```python
from build123d import *

# Parameters (mm, degrees)
F0_R           = 6.35
F1_DEPTH       = 25.4
F2_R           = 6.35
F3_DEPTH       = 13.716
F5_DEPTH       = 7.493
F6_DEPTH       = 5.08
F8_D           = 2.921
F8_CBORE_D     = 4.699
F8_CBORE_DEPTH = 10.922
F9_DEPTH       = 10.922
F10_DEPTH      = 17.907


with BuildPart() as f1:
    # F0 (on Front) → F1 (new body)
    with BuildSketch(Plane.XZ):
        with BuildLine():
            Line((0, -13.589), (17.1026142738, -13.589))
            ThreePointArc((17.1026142738, -13.589), (0, 21.844), (-17.1026142738, -13.589))
            Line((-17.1026142738, -13.589), (0, -13.589))
        make_face()
        Circle(F0_R, mode=Mode.SUBTRACT)
    extrude(amount=F1_DEPTH)

    # F2 (on face) → F3 (cut)
    with BuildSketch(Plane(origin=(0, 0, 0), x_dir=(-1, 0, 0), z_dir=(0, 1, 0))):
        with BuildLine():
            Line((-3.2512, 21.6006952333), (-3.2512, 15.5385109827))
            ThreePointArc((-3.2512, 15.5385109827), (-15.6500961726, 2.6627269459), (-8.2069911661, -13.589))
            Line((-8.2069911661, -13.589), (8.2069911661, -13.589))
            ThreePointArc((8.2069911661, -13.589), (15.6500961726, 2.6627269459), (3.2512, 15.5385109827))
            Line((3.2512, 15.5385109827), (3.2512, 21.6006952333))
            ThreePointArc((3.2512, 21.6006952333), (0, 21.844), (-3.2512, 21.6006952333))
        make_face()
        Circle(F2_R, mode=Mode.SUBTRACT)
    extrude(amount=-F3_DEPTH, mode=Mode.SUBTRACT)

    # F4 (on face) → F5 (cut)
    with BuildSketch(Plane(origin=(0, 0, 0), x_dir=(-1, 0, 0), z_dir=(0, 1, 0))):
        with BuildLine():
            Line((-17.1026142738, -13.589), (-8.2069911661, -13.589))
            ThreePointArc((-8.2069911661, -13.589), (-15.6500961726, 2.6627269459), (-3.2512, 15.5385109827))
            Line((-3.2512, 15.5385109827), (-3.2512, 16.129))
            Line((-3.2512, 16.129), (-14.731452576, 16.129))
            ThreePointArc((-14.731452576, 16.129), (-16.3464246709, 14.4898149222), (-17.78, 12.6898359327))
            Line((-17.78, 12.6898359327), (-17.78, -12.6898359327))
            ThreePointArc((-17.78, -12.6898359327), (-17.44710058, -13.1437824598), (-17.1026142738, -13.589))
        make_face()
        with BuildLine():
            Line((-8.2069911661, -13.589), (0, -13.589))
            Line((0, -13.589), (17.78, -13.589))
            Line((17.78, -13.589), (17.78, 16.129))
            Line((17.78, 16.129), (-3.2512, 16.129))
            Line((-3.2512, 16.129), (-3.2512, 15.5385109827))
            ThreePointArc((-3.2512, 15.5385109827), (-15.6500961726, 2.6627269459), (-8.2069911661, -13.589))
        make_face()
    extrude(amount=-F5_DEPTH, mode=Mode.SUBTRACT)

    # F6 (cut): faces of the model
    f6_faces = [f1.faces().sort_by_distance(p)[0] for p in [
        (7.5018293791, 0, 18.2089166426),
        (-7.5018293791, 0, 18.2089166426),
    ]]
    extrude(f6_faces, amount=-F6_DEPTH, mode=Mode.SUBTRACT)

    # F8 (through all)
    with Locations(Plane.XZ.offset(25.4)):
        with Locations((-14.2875, -9.1525132509), (-14.2875, 12.3104867491), (14.2875, 12.3104867491), (14.2875, -9.1525132509)):
            CounterBoreHole(F8_D / 2, F8_CBORE_D / 2, F8_CBORE_DEPTH)

    # F7 (on face) → F9 (cut)
    with BuildSketch(Plane.XZ.offset(25.4)):
        with BuildLine():
            Line((-12.827, -13.589), (-11.938, -13.589))
            Line((-11.938, -13.589), (-11.938, -9.1525132509))
            ThreePointArc((-11.938, -9.1525132509), (-12.1990496422, -8.0761650949), (-12.9241888511, -7.239))
            Line((-12.9241888511, -7.239), (-13.6989384625, -7.239))
            ThreePointArc((-13.6989384625, -7.239), (-13.8035807397, -7.0374139258), (-13.9052567889, -6.8343155938))
            ThreePointArc((-13.9052567889, -6.8343155938), (-15.8077088385, -7.3611128665), (-16.637, -9.1525132509))
            Line((-16.637, -9.1525132509), (-16.637, -13.589))
            Line((-16.637, -13.589), (-15.748, -13.589))
            Line((-15.748, -13.589), (-15.748, -9.1525132509))
            ThreePointArc((-15.748, -9.1525132509), (-14.2875, -7.6920132509), (-12.827, -9.1525132509))
            Line((-12.827, -9.1525132509), (-12.827, -13.589))
        make_face()
        with BuildLine():
            ThreePointArc((12.827, -9.1525132509), (14.2875, -7.6920132509), (15.748, -9.1525132509))
            Line((15.748, -9.1525132509), (15.748, -13.589))
            Line((15.748, -13.589), (16.637, -13.589))
            Line((16.637, -13.589), (16.637, -9.1525132509))
            ThreePointArc((16.637, -9.1525132509), (15.8077088385, -7.3611128665), (13.9052567889, -6.8343155938))
            ThreePointArc((13.9052567889, -6.8343155938), (13.8035807397, -7.0374139258), (13.6989384625, -7.239))
            Line((13.6989384625, -7.239), (12.9241888511, -7.239))
            ThreePointArc((12.9241888511, -7.239), (12.1990496422, -8.0761650949), (11.938, -9.1525132509))
            Line((11.938, -9.1525132509), (11.938, -13.589))
            Line((11.938, -13.589), (12.827, -13.589))
            Line((12.827, -13.589), (12.827, -9.1525132509))
        make_face()
    extrude(amount=-F9_DEPTH, mode=Mode.SUBTRACT)

    # F7 (on face) → F10 (cut)
    with BuildSketch(Plane.XZ.offset(25.4)):
        with BuildLine():
            Line((-15.748, -13.589), (-12.827, -13.589))
            Line((-12.827, -13.589), (-12.827, -9.1525132509))
            ThreePointArc((-12.827, -9.1525132509), (-14.2875, -7.6920132509), (-15.748, -9.1525132509))
            Line((-15.748, -9.1525132509), (-15.748, -13.589))
        make_face()
        with BuildLine():
            Line((15.748, -13.589), (15.748, -9.1525132509))
            ThreePointArc((15.748, -9.1525132509), (14.2875, -7.6920132509), (12.827, -9.1525132509))
            Line((12.827, -9.1525132509), (12.827, -13.589))
            Line((12.827, -13.589), (15.748, -13.589))
        make_face()
    extrude(amount=-F10_DEPTH, mode=Mode.SUBTRACT)


solid = f1.part
```
The model under review builds one solid part; all positions refer to its coordinate system, in mm. A direction names the side the tool comes from. Round coordinates to 2 decimals unless told otherwise and drop trailing zeros. Loops run counter-clockwise (first coordinate to the right, second up) from the corner with the lowest first, then second, coordinate; pieces in that order, holes last. Notation, with made-up numbers: (-4.5, 17.25) -> (45.5, 17.25) arc R30 cw to (45.5, 55.25) -> close; hole circle Ø1 at (14.25, -30.5). An arc over 180 degrees is marked (long way). Answer as a JSON object with one key per item and string values. Group by question number.
1) For faces 1 (the face through (13, -14.478, 11)), 2 (the face through (12.827, -11, -11)), 3 (the face through (-9, -6, 16.129)), list the 3-axis set-ups (+Z, -Z, +X, -X, +Y, -Y) from which the entire face can be reached by the end or side of a thin tool; tool diameter is ignored.
2) We need section B-B on y = -6.25. Write out the cut boundary in (x, z).
3) Mouldability with a two-part tool opening along X and no side actions: class faces 4 (the face through (-12.75, -14.478, 11.82)), 5 (the face through (19, 0, 0)), 6 (the face through (0.686, -15.344, 21.833)) as released by +X, released by -X, zero draft, split by the parting line, or undercut.
4) We need section D-D on y = -10.5. Give the number of separate pieces and of enclosed holes in the cut face, then the cut area to 3 significant figures.
5) For line 1 (X direction, y = -8.5, z = -11); line 2 (X direction, y = -18.25, z = -8); line 3 (X direction, y = -23.5, z = -9.5), list the stretches that pass through material, from the lowest coordinate up. Write a range as [from, to].
6) We need section A-A on z = 0. Write out the cut boundary in (x, y) (3 decimals).
7) For pin 1 Ø16 at (x, z) = (-2.5, -1.5) entering from +Y; pin 2 Ø6 at (x, z) = (11, 20) entering from +Y; pin 3 Ø4.5 at (x, z) = (-11, -11) entering from +Y, all flat-tipped, find the tip position at first contact; note any pin that passes through.
8) We need section C-C on x = 0. Write out the cut boundary in (y, z), then the cut area to 3 significant figures.
Result set:
{
 "1": {"face 1": "-Y", "face 2": "-Z, +Y, -Y", "face 3": "-Z, +X, -X, +Y"},
 "2": {"outline": "(-17.78, -12.69) -> (-17.78, 12.69) arc R21.84 ccw to start; (-14.73, 16.13) -> (-3.25, 16.13) -> (-3.25, 21.6) arc R21.84 ccw to start; (3.25, 16.13) -> (14.73, 16.13) arc R21.84 ccw to (3.25, 21.6) -> close; (17.78, -12.69) arc R21.84 ccw to (17.78, 12.69) -> close"},
 "3": {"face 4": "undercut", "face 5": "zero draft", "face 6": "split by the parting line"},
 "4": {"separate pieces": "4", "enclosed holes": "2", "area": "452 mm²"},
 "5": {"line 1": "[-18.87, -15.75], [-12.83, -11.45], [11.45, 12.83], [15.75, 18.87]", "line 2": "[-20.33, -16.33], [-12.24, 12.24], [16.33, 20.33]", "line 3": "[-19.67, -16.64], [-11.94, 11.94], [16.64, 19.67]"},
 "6": {"outline": "(-21.844, -25.4) -> (-6.35, -25.4) -> (-6.35, -13.716) -> (-15.875, -13.716) -> (-15.875, -7.493) -> (-17.78, -7.493) -> (-17.78, 0) -> (-21.844, 0) -> close; (6.35, -25.4) -> (21.844, -25.4) -> (21.844, 0) -> (17.78, 0) -> (17.78, -7.493) -> (15.875, -7.493) -> (15.875, -13.716) -> (6.35, -13.716) -> close"},
 "7": {"pin 1": "y = -13.72", "pin 2": "y = -5.08", "pin 3": "y = -7.49"},
 "8": {"outline": "(-25.4, -13.59) -> (-13.72, -13.59) -> (-13.72, -6.35) -> (-25.4, -6.35) -> close; (-25.4, 6.35) -> (-13.72, 6.35) -> (-13.72, 21.84) -> (-25.4, 21.84) -> close", "area": "266 mm²"}
}
